Autodesk Fusion 360 part; units mm, degrees
sketch "Sketch1" plane through (0, 0, 0) normal (0, 1, 0) x (1, 0, 0)
  line L0 (50.8, 6.35) -> (-50.8, 6.35)
  line L1 (-50.8, 6.35) -> (-50.8, -6.35)
  line L2 (-50.8, -6.35) -> (50.8, -6.35)
  line L3 (50.8, -6.35) -> (50.8, 6.35)
  line L4 (50.8, 6.35) -> (-50.8, -6.35) construction
  line L5 (-50.8, 6.35) -> (50.8, -6.35) construction
  dimension "d1" = 101.6
  dimension "d2" = 12.7
extrude "Extrude1" add sketch "Sketch1" along normal mid plane 50.8
sketch "Sketch2" plane through (0, 0, 0) normal (0, 1, 0) x (1, 0, 0)
  line L0 (50.8, -6.35) -> (-50.8, -6.35)
  line L1 (-25.4, -6.35) -> (26.3955, -30.5026)
  dimension "d5" = 25.4
  dimension "d6" = 25
  dimension "d7" = 57.15
ref_plane "WorkPlane1" through (26.3955, 0, 30.5026) normal (0.9063, 0, 0.4226) x (0, 1, 0)
sketch "Sketch3" plane through (26.3955, 0, 30.5026) normal (0.9063, 0, 0.4226) x (0, 1, 0)
  circle A0 centre (0, 0) radius 6.35
  circle A1 centre (0, 0) radius 9.525
  line L0 (-9.525, 0) -> (-9.525, -26.6495)
  line L1 (-9.525, -26.6495) -> (9.525, -26.6495)
  line L2 (9.525, -26.6495) -> (9.525, 0)
  line L3 (25.4, -26.6495) -> (-25.4, -26.6495)
  dimension "d9" = 12.7
  dimension "d10" = 19.05
extrude "Extrude2" add sketch "Sketch3" along normal up to surface contours A0 | A1 | A1 L0 L1 L2 L3 end surface through (-50.8, 0, 6.35) normal (0, 0, 1) offset 0
extrude "Extrude3" cut sketch "Sketch3" against normal blind 25.4 contours A0
fillet "Fillet1" radius 6.35 4 edges at (-50.8, -25.4, 0) (-50.8, 25.4, 0) (50.8, 25.4, 0) (50.8, -25.4, 0)
Check sheet for the modelled part. Datum: model origin and axes. Units: mm. A direction names the side the tool comes from. Give positions to 0.01 mm unless a question says otherwise; leave off trailing zeros. Loops run counter-clockwise (first coordinate to the right, second up) from the corner with the lowest first, then second, coordinate; pieces in that order, holes last. Notation, with made-up numbers: M 44,56.5 L 99,56.5 A10 ccw 99,65.5 Z; hole C 56.25,-28 d1. An arc over 180 degrees is marked long. Return JSON: item names as keys, results as strings. Group by question number.
1. Cross-section at B-B on y = 4.5. Record the boundary of the cut face in (x, z).
2. Tool access check on faces 1 (the flat face through (11, -9.525, 12)), 2 (the cylindrical face through (-12.322, 0.209, 22.956)). Record the directions out of +Z, -Z, +X, -X, +Y, -Y that give a thin tool (end or side, any length) a straight path to the whole face; none if there is none.
3. Go/stop test with flat-tipped pins: pin 1 (15 mm diameter, centred on x = -12.5, y = -12.5, fed in from +Z); pin 2 (8 mm diameter, centred on x = 7, z = 12, fed in from +Y) (3 decimals); pin 3 (10 mm diameter, centred on x = -11, y = 3, fed in from +Z). Record where each tip stops, or that it passes through.
4. Thickness scan on L1, parallel to Y at x = 20, z = 28; L2, parallel to Z at x = 34, y = 19.5. Record the ranges inside material, lowest first.
5. Cross-section at D-D on y = 21.5. Record the boundary of the cut face in (x, z).
6. Cross-section at A-A on x = 33.5. Record the boundary of the cut face in (y, z) (3 decimals).
7. Cross-section at C-C on y = 11. Record the boundary of the cut face in (x, z).
8. Mould release check, pull along Z, two halves, no side actions. Record for faces 3 (the cylindrical face through (-48.99, -23.49, 0.09)), 4 (the cylindrical face through (16.07, 5.87, 23.01)), 5 (the flat face through (3.338, -0.089, 19.849)), 6 (the flat face through (-1, 11, 6.35)): released by +Z, released by -Z, zero draft, split by the parting line, or undercut.
Return value:
{
 "1": {"outline": "M -50.8,-6.35 L 50.8,-6.35 L 50.8,6.35 L 37.66,6.35 L 28.29,26.44 L 5.27,15.71 L 1.48,23.83 L 24.5,34.56 L 22.85,38.11 L -45.26,6.35 L -50.8,6.35 Z"},
 "2": {"face 1": "+Z, +X, -X, -Y", "face 2": "+Z, -X"},
 "3": {"pin 1": "z = 22.28", "pin 2": "y = 9.525", "pin 3": "z = 25.67"},
 "4": {"L1": "-9.52 to -6.34, 6.34 to 9.52", "L2": "-6.35 to 6.35"},
 "5": {"outline": "M -50.31,-6.35 L 50.31,-6.35 L 50.31,6.35 L -50.31,6.35 Z"},
 "6": {"outline": "M -25.4,-6.35 L 25.4,-6.35 L 25.4,6.35 L 9.525,6.35 L 9.525,15.267 L -9.525,15.267 L -9.525,6.35 L -25.4,6.35 Z"},
 "7": {"outline": "M -50.8,-6.35 L 50.8,-6.35 L 50.8,6.35 L -50.8,6.35 Z"},
 "8": {"face 3": "zero draft", "face 4": "undercut", "face 5": "undercut", "face 6": "released by +Z"}
}
